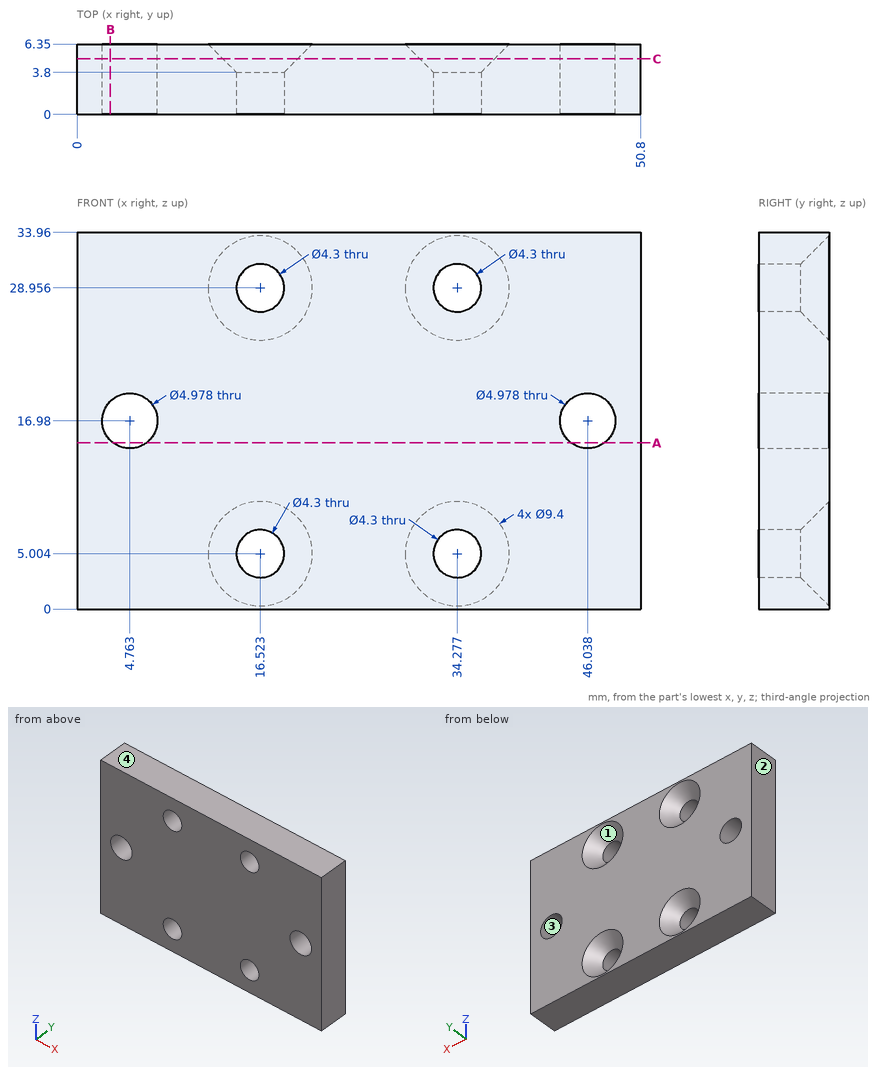
Could you check a few things on this drawing? It's one solid part, dimensions in mm from its lowest x, y, z. Coordinates: 2 decimals unless noted, no trailing zeros. Loops run counter-clockwise (first coordinate to the right, second up) from the corner with the lowest first, then second, coordinate; pieces in that order, holes last.
1. Imagine slicing it at B-B (x = 3). Please give me the cut outline in (y, z).
2. For P1, Ø3, axis at x = 40.5, y = 1, coming from the -Z side; P2, Ø7, axis at x = 34.28, z = 5, coming from the +Y side (1 decimal); P3, Ø5, axis at x = 16.52, z = 5, coming from the +Y side (1 decimal); P4, Ø4, axis at x = 34.28, z = 28.96, coming from the +Y side, each with a flat end and sliding along its axis, tell me the tip position at first contact or that it passes through.
3. Imagine slicing it at C-C (y = 5). Give the number of separate pieces and of enclosed holes in the cut face, and give its area (4 significant figures).
4. We'd pull the mould along Z, two halves only. Please class the marked faces 1, 2, 3 and 4: released by +Z, released by -Z, zero draft, split by the parting line, or undercut.
5. Imagine slicing it at A-A (z = 15). Please give me the cut outline in (x, y), and give its area (3 significant figures).
6. I need wall thicknesses on L1, parallel to Z at x = 19, y = 6.25 (1 decimal); L2, parallel to X at y = 5.75, z = 2 (1 decimal); L3, parallel to Z at x = 15, y = 1.75 (1 decimal). Which ranges of each line are inside material? Lowest first, please.
Computed values:
1. outline: (0, 0) - (6.35, 0) - (6.35, 15.22) - (0, 15.22) - close; (0, 18.74) - (6.35, 18.74) - (6.35, 33.96) - (0, 33.96) - close
2. P1: stops at z = 0
2. P2: stops at y = 5.2
2. P3: stops at y = 4.2
2. P4: passes through
3. separate pieces: 1
3. enclosed holes: 6
3. area: 1,545 mm2
4. face 1: undercut
4. face 2: zero draft
4. face 3: undercut
4. face 4: released by +Z
5. outline: (0, 0) - (3.25, 0) - (3.25, 6.35) - (0, 6.35) - close; (6.27, 0) - (44.53, 0) - (44.53, 6.35) - (6.27, 6.35) - close; (47.55, 0) - (50.8, 0) - (50.8, 6.35) - (47.55, 6.35) - close
5. area: 284 mm2
6. L1: z = 0 to 1.1, 8.9 to 25.1, 32.8 to 34
6. L2: x = 0 to 13.7, 19.3 to 31.5, 37.1 to 50.8
6. L3: z = 0 to 3.5, 6.5 to 27.4, 30.5 to 34
